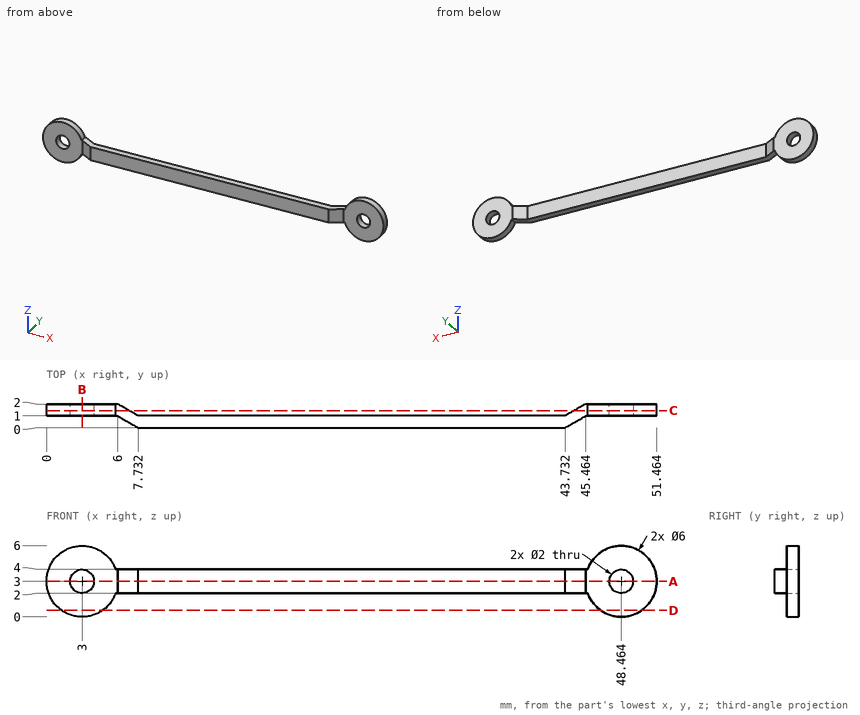
Geometry check sheet. Reference: drawing and pictorial views, mm from the part's lowest x, y, z. Round coordinates to 2 decimals unless told otherwise and drop trailing zeros. Order: outer loops, then holes, each group sorted by start corner. A loop starts at its lowest first (then second) coordinate and runs counter-clockwise, first axis right, second up. Notation, with made-up numbers: (56.25, 21) - (66.25, 21) arc R13 ccw to (66.25, 31) - close; hole circle Ø5 at (-21, 34.5). An arc over 180 degrees is marked (long way). Write item = value, one per line.
Q1. Section check A-A (z = 3). Record the boundary of the cut face in (x, y).
Computed:
outline = (0, 1) - (2, 1) - (2, 2) - (0, 2) - close; (4, 1) - (6, 1) - (7.73, 0) - (43.73, 0) - (45.46, 1) - (47.46, 1) - (47.46, 2) - (45.46, 2) - (43.73, 1) - (7.73, 1) - (6, 2) - (4, 2) - close; (49.46, 1) - (51.46, 1) - (51.46, 2) - (49.46, 2) - close
Q2. Thickness scan on line 1 along X through (y, z) = (1.65, 3) (1 decimal); line 2 along X through (y, z) = (1.6, 3) (1 decimal); line 3 along Z through (x, y) = (3, 1.25). Record the ranges inside material, lowest first.
Computed:
line_1 = 0 to 2, 4 to 6.6, 44.9 to 47.5, 49.5 to 51.5
line_2 = 0 to 2, 4 to 6.7, 44.8 to 47.5, 49.5 to 51.5
line_3 = 0 to 2, 4 to 6
Q3. Section check D-D (z = 0.55). Record the boundary of the cut face in (x, y).
Computed:
outline = (1.27, 1) - (4.73, 1) - (4.73, 2) - (1.27, 2) - close; (46.73, 1) - (50.2, 1) - (50.2, 2) - (46.73, 2) - close
Q4. Go/stop test with flat-tipped pins: pin 1 (1.8 mm diameter, centred on x = 48, z = 2, fed in from -Y); pin 2 (2 mm diameter, centred on x = 21.5, z = 3, fed in from +Y). Record where each tip stops, or that it passes through.
Computed:
pin_1 = 1
pin_2 = 1
Q5. Section check C-C (y = 1.45). Record the boundary of the cut face in (x, z), and give its area (3 significant figures).
Computed:
outline = (5.83, 2) - (6.95, 2) - (6.95, 4) - (5.83, 4) arc R3 ccw (long way) to start; (44.51, 2) - (45.64, 2) arc R3 ccw (long way) to (45.64, 4) - (44.51, 4) - close; hole circle Ø2 at (3, 3); hole circle Ø2 at (48.46, 3)
area = 54.3 mm^2
Q6. Section check B-B (x = 3). Record the boundary of the cut face in (y, z), and give its area (3 significant figures).
Computed:
outline = (1, 0) - (2, 0) - (2, 2) - (1, 2) - close; (1, 4) - (2, 4) - (2, 6) - (1, 6) - close
area = 4.00 mm^2
